Geometry check sheet. Reference: the model listing, model coordinates, mm. Face numbers are marked on the shaded views. A direction names the side the tool comes from. Round coordinates to 2 decimals unless told otherwise and drop trailing zeros. Write each loop counter-clockwise with the first axis right and the second up, starting at its lowest first coordinate (ties: lowest second). Pieces come first, ordered by that corner, then holes. Notation, with made-up numbers: (52.5, 81.5) -> (95.5, 81.5) arc R23 ccw to (95.5, 97.5) -> close; hole circle Ø8 at (28, 31.5). An arc over 180 degrees is marked (long way). Use a Markdown table: item, result.
```python
from build123d import *
from build123d.topology import SkipClean

# Parameters (mm, degrees)
BOSS_EXTRUDE1_START = 30
BOSS_EXTRUDE1_DEPTH = 30
CIRPATTERN1_COUNT   = 8
SKETCH3_R           = 8
BOSS_EXTRUDE2_DEPTH = 30


with BuildPart() as part:
    # Sketch1 → Revolve1 (revolve)
    with BuildSketch(Plane(origin=(0, 0, 0), x_dir=(0, 0, -1), z_dir=(1, 0, 0)), mode=Mode.PRIVATE) as revolve1_sk:
        with BuildLine():
            Line((0, 0), (0, 78))
            Line((0, 78), (-3, 78))
            Line((-3, 78), (-3, 13))
            Line((-3, 13), (-20, 13))
            ThreePointArc((-20, 13), (-27.071067812, 10.071067812), (-30, 3))
            Line((-30, 3), (-30, 0))
            Line((-30, 0), (0, 0))
        make_face()
    revolve(revolve1_sk.sketch.rotate(Axis((0, 0, 30), (0, 0, -1)), 90), axis=Axis((0, 0, 30), (0, 0, -1)))

    # Sketch2 → Boss-Extrude1 (add)
    with BuildSketch(Plane.XY.offset(3).offset(BOSS_EXTRUDE1_START)):
        with BuildLine():
            ThreePointArc((-21.213203436, 21.213203436), (-19.654544502, 22.664926217), (-17.996806645, 24.002394684))
            ThreePointArc((-17.996806645, 24.002394684), (-15.924246169, 56.688991773), (9.42496759, 77.42848304))
            ThreePointArc((9.42496759, 77.42848304), (4.721139844, 77.856989658), (0, 78))
            ThreePointArc((0, 78), (-21.603078805, 53.7144317), (-21.213203436, 21.213203436))
        make_face()
    boss_extrude1 = extrude(amount=-BOSS_EXTRUDE1_DEPTH)

    # CirPattern1: Boss-Extrude1 ×8 about axis
    with SkipClean():  # the faces are left unmerged after this step: merging them gives an invalid solid
        cirpattern1_axis = Axis((0, 0, 0), (0, 0, 1))
        for i in range(1, CIRPATTERN1_COUNT):
            add(boss_extrude1.rotate(cirpattern1_axis, i * 360 / CIRPATTERN1_COUNT))

    # Sketch3 → Boss-Extrude2 (add)
    with SkipClean():  # the faces are left unmerged after this step: merging them gives an invalid solid
        with BuildSketch(Plane(origin=(0, 0, 0), x_dir=(-1, 0, 0), z_dir=(0, 0, -1))):
            with Locations(Location((0, 0, 0), (0, 0, 180))):
                Circle(SKETCH3_R)
        extrude(amount=BOSS_EXTRUDE2_DEPTH)


solid = part.part
```
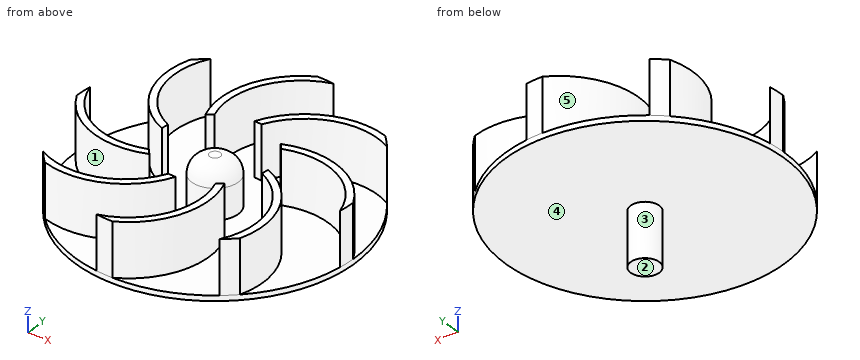
(1) Thickness scan on line 1 (X direction, y = 38.5, z = 30); line 2 (Y direction, x = -36.5, z = 29.5); line 3 (Y direction, x = -49, z = 28.5). Record the ranges inside material, lowest first.
A:
| item | result |
|---|---|
| line 1 | x = -57.22 to -53.21, -24.45 to -20.44, 4.78 to 9.83 |
| line 2 | y = -57.05 to -53.02, -24.42 to -20.42, 3.43 to 8.27 |
| line 3 | y = -56.66 to -52.6, -23.07 to -18.94, 15.32 to 23.07, 59.69 to 60.69 |
(2) Release check for a two-part mould opening along Y. For the marked faces 3, 4 and 5 record: +Y half, -Y half, draft (parallel to the pull), parting line (faces both ways), or undercut.
A:
| item | result |
|---|---|
| face 3 | parting line |
| face 4 | draft |
| face 5 | undercut |
(3) Section check A-A on z = 6. State how many separate pieces and enclosed holes the cut face has, plus the area to 3 significant figures.
A:
| item | result |
|---|---|
| separate pieces | 9 |
| enclosed holes | 0 |
| area | 2,670 mm2 |
(4) Section check B-B on x = -50.5. Record the cut outline in (y, z).
A:
| item | result |
|---|---|
| outline | (-59.45, 0) -> (59.45, 0) -> (59.45, 33) -> (56.31, 33) -> (56.31, 3) -> (26.45, 3) -> (26.45, 33) -> (17.57, 33) -> (17.57, 3) -> (-18.49, 3) -> (-18.49, 33) -> (-22.67, 33) -> (-22.67, 3) -> (-52.29, 3) -> (-52.29, 33) -> (-56.38, 33) -> (-56.38, 3) -> (-59.45, 3) -> close |
(5) Access from +Z, -Z, +X, -X, +Y, -Y to the whole of each face (thin tool, end or side, straight path). Record for the marked faces 1 and 2.
A:
| item | result |
|---|---|
| face 1 | +Z |
| face 2 | -Z, +X, -X, +Y, -Y |
(6) Section check C-C on y = -37. Record the cut outline in (x, z), plus the area to 3 significant figures.
A:
| item | result |
|---|---|
| outline | (-68.67, 0) -> (68.67, 0) -> (68.67, 3) -> (57.1, 3) -> (57.1, 33) -> (53.08, 33) -> (53.08, 3) -> (24.44, 3) -> (24.44, 33) -> (20.44, 33) -> (20.44, 3) -> (-3.75, 3) -> (-3.75, 33) -> (-8.64, 33) -> (-8.64, 3) -> (-68.67, 3) -> close |
| area | 799 mm2 |
(7) Gauge pin test, flat ends, axial feed: pin 1 Ø6 at (x, z) = (-58, 6.5) entering from -Y; pin 2 Ø1.8 at (x, y) = (-0.5, 0.5) entering from +Z; pin 3 Ø6 at (x, z) = (14, 18) entering from +Y. Record the tip position at first contact, or that the pin passes through.
A:
| item | result |
|---|---|
| pin 1 | stops at y = -55.2 |
| pin 2 | stops at z = 30 |
| pin 3 | stops at y = 50.14 |
